from build123d import *

# Parameters (mm, degrees)
F0_R     = 1.5
F1_DEPTH = 3
F3_DEPTH = 2
F7_R     = 1.5
F8_DEPTH = 3


with BuildPart() as f1:
    # F0 (on Top) → F1 (new body)
    with BuildSketch(Plane.XY):
        with BuildLine():
            Line((8, 0), (8, 5.5929704658))
            ThreePointArc((8, 5.5929704658), (1.25, 20), (8, 34.4070295342))
            Line((8, 34.4070295342), (8, 75))
            Line((8, 75), (20, 75))
            Line((20, 75), (32, 75))
            Line((32, 75), (32, 34.4070295342))
            ThreePointArc((32, 34.4070295342), (38.75, 20), (32, 5.5929704658))
            Line((32, 5.5929704658), (32, 0))
            Line((32, 0), (43, 0))
            Line((43, 0), (43, 78))
            Line((43, 78), (20, 78))
            Line((20, 78), (-3, 78))
            Line((-3, 78), (-3, 0))
            Line((-3, 0), (8, 0))
        make_face()
        with Locations((4, 4)):
            Circle(F0_R, mode=Mode.SUBTRACT)
        with Locations((4, 36)):
            Circle(F0_R, mode=Mode.SUBTRACT)
        with Locations((36, 4)):
            Circle(F0_R, mode=Mode.SUBTRACT)
        with Locations((36, 36)):
            Circle(F0_R, mode=Mode.SUBTRACT)
    extrude(amount=-F1_DEPTH)

    # F2 (on face) → F3 (join)
    with BuildSketch(Plane(origin=(-3, 0, 0), x_dir=(0, -1, 0), z_dir=(-1, 0, 0))):
        Polygon((-78, -3), (0, -3), (0, 2), (-75, 22), (-78, 22), align=None)
    extrude(amount=F3_DEPTH)

    # F6: F1 across plane


with BuildPart() as f1_1:
    add(f1.part)
    add(f1.part.mirror(Plane.YZ.offset(20)))

    # F7 (on face) → F8 (join, through all)
    with BuildSketch(Plane(origin=(0, 78, 0), x_dir=(-1, 0, 0), z_dir=(0, 1, 0))):
        Polygon((-45, 22), (-45, -3), (5, -3), (5, 22), (3, 22), (-20, 13.8037335128), (-43, 22), align=None)
        with Locations((-36.5411415696, 13.6936744675)):
            Circle(F7_R, mode=Mode.SUBTRACT)
        with Locations((-3.4588584304, 13.6936744675)):
            Circle(F7_R, mode=Mode.SUBTRACT)
    extrude(amount=-F8_DEPTH)


solid = f1_1.part
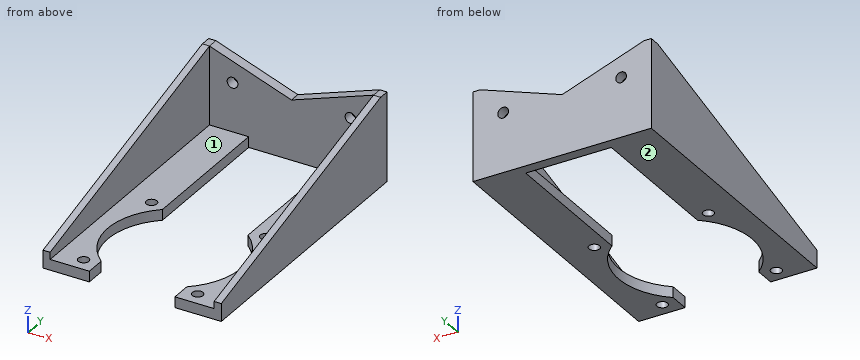
The listing builds one solid part. Answer for the finished solid, in the listing's coordinates (mm). Face numbers are marked on the shaded views. A direction names the side the tool comes from. Coordinates: 2 decimals unless noted, no trailing zeros. Loops run counter-clockwise (first coordinate to the right, second up) from the corner with the lowest first, then second, coordinate; pieces in that order, holes last. Notation, with made-up numbers: M 81,66.25 L 109,66.25 A11 cw 109,84.25 Z; hole C -16,34 d3. An arc over 180 degrees is marked long. Answer in a Markdown table with one row per item.
1) Find section B-B (y = 45). Determine the outline of the cut face in (x, z).
Answers below:
| item | result |
|---|---|
| outline | M -5,-3 L 8,-3 L 8,0 L -3,0 L -3,14 L -5,14 Z; M 32,-3 L 45,-3 L 45,14 L 43,14 L 43,0 L 32,0 Z |
2) Find section D-D (z = 8). Determine the outline of the cut face in (x, y), then the cut area to 3 significant figures.
Answers below:
| item | result |
|---|---|
| outline | M -5,22.5 L -3,22.5 L -3,75 L 43,75 L 43,22.5 L 45,22.5 L 45,78 L -5,78 Z |
| area | 360 mm^2 |
3) Find the intervals of material crossed by probe 1 along X at (y, z) = (74, 12.25); probe 2 along Y at (x, z) = (4, -1.4); probe 3 along Y at (x, z) = (31, 8), in increasing order.
Answers below:
| item | result |
|---|---|
| probe 1 | -5 to -3, 43 to 45 |
| probe 2 | 0 to 2.5, 5.5 to 10.22, 29.78 to 34.5, 37.5 to 78 |
| probe 3 | 75 to 78 |
4) Find section A-A (y = 36). Determine the outline of the cut face in (x, z).
Answers below:
| item | result |
|---|---|
| outline | M -5,-3 L 2.5,-3 L 2.5,0 L -3,0 L -3,11.6 L -5,11.6 Z; M 5.5,-3 L 8,-3 L 8,0 L 5.5,0 Z; M 32,-3 L 34.5,-3 L 34.5,0 L 32,0 Z; M 37.5,-3 L 45,-3 L 45,11.6 L 43,11.6 L 43,0 L 37.5,0 Z |
5) Find section C-C (z = -1.25). Determine the outline of the cut face in (x, y).
Answers below:
| item | result |
|---|---|
| outline | M -5,0 L 8,0 L 8,5.59 A18.75 cw 8,34.41 L 8,75 L 32,75 L 32,34.41 A18.75 cw 32,5.59 L 32,0 L 45,0 L 45,78 L -5,78 Z; hole C 4,4 d3; hole C 4,36 d3; hole C 36,4 d3; hole C 36,36 d3 |
6) Which of the six approach directions +Z, -Z, +X, -X, +Y, -Y give full straight-line access (tool end or side, diameter ignored) to the marked faces 1 and 2?
Answers below:
| item | result |
|---|---|
| face 1 | +Z, -Y |
| face 2 | -Z, +X, -X, +Y, -Y |
7) Given pin 1 (1.5 mm diameter, centred on x = 34.5, y = 32.5, fed in from +Z); pin 2 (12 mm diameter, centred on x = 2.5, y = 56, fed in from +Z); pin 3 (1.5 mm diameter, centred on x = 1.5, z = 14.5, fed in from -Y), each flat-ended and moving along its own axis, determine where each tip first touches the part or whether it passes through.
Answers below:
| item | result |
|---|---|
| pin 1 | z = 0 |
| pin 2 | z = 17.57 |
| pin 3 | y = 75 |
